Geometry check sheet. Reference: drawing and pictorial views, mm from the part's lowest x, y, z. Give positions to 0.01 mm unless a question says otherwise; leave off trailing zeros. Order: outer loops, then holes, each group sorted by start corner. A loop starts at its lowest first (then second) coordinate and runs counter-clockwise, first axis right, second up. Notation, with made-up numbers: (55, -37.75) - (59, -37.75) arc R19 cw to (59, -9.75) - close; hole circle Ø6 at (48.5, 30). An arc over 180 degrees is marked (long way). Answer as a JSON object with one key per item and string values.
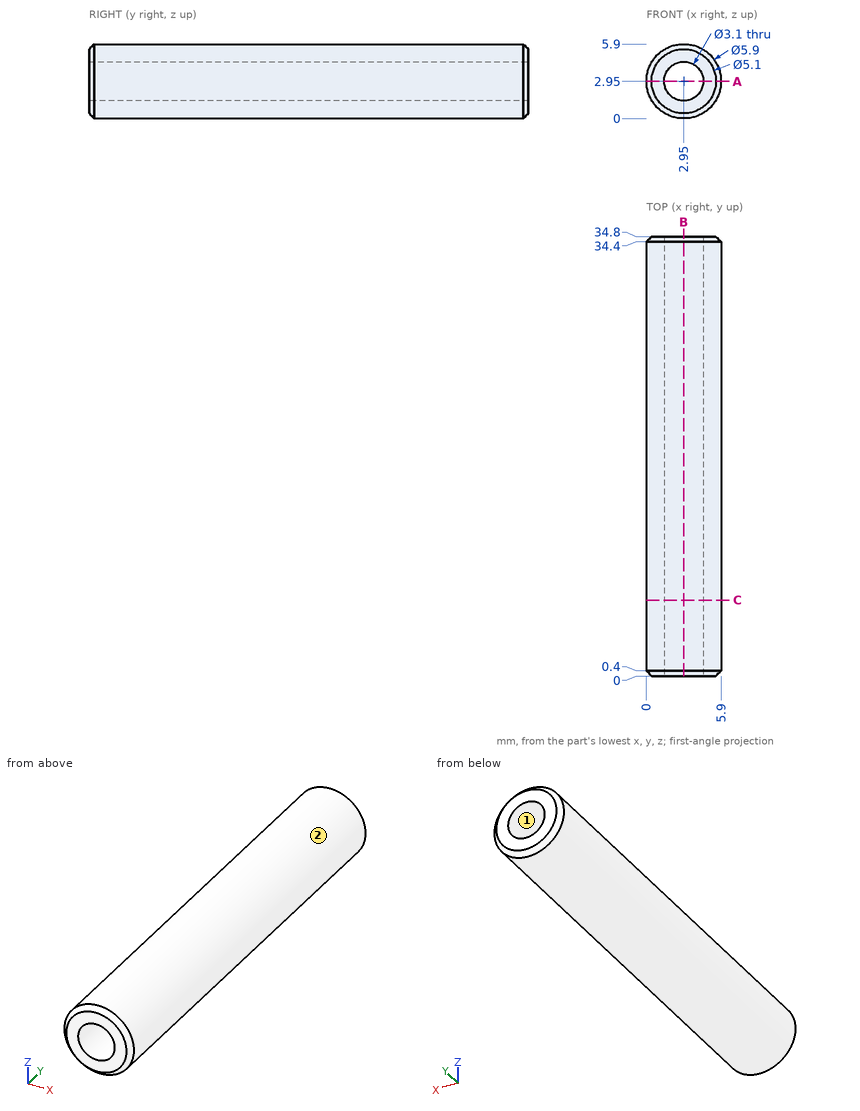
(1) Release check for a two-part mould opening along Z. For the marked faces 1 and 2 record: pulls with the +Z half, pulls with the -Z half, needs draft (parallel to the pull), parting line crosses it, or undercut.
Computed values:
{"face 1": "undercut", "face 2": "parting line crosses it"}
(2) Section check B-B (x = 2.95). Record the cut outline in (y, z), then the cut area to 3 significant figures.
Computed values:
{"outline": "(0, 0.4) - (0.4, 0) - (34.4, 0) - (34.8, 0.4) - (34.8, 1.4) - (0, 1.4) - close; (0, 4.5) - (34.8, 4.5) - (34.8, 5.5) - (34.4, 5.9) - (0.4, 5.9) - (0, 5.5) - close", "area": "97.1 mm²"}
(3) Material ranges on line 1 along X through (y, z) = (10.5, 2.95); line 2 along Z through (x, y) = (3.1, 22); line 3 along Z through (x, y) = (2.1, 18), recorded low to high. Write a range as [from, to].
Computed values:
{"line 1": "x = [0, 1.4], [4.5, 5.9]", "line 2": "z = [0, 1.41], [4.49, 5.9]", "line 3": "z = [0.13, 1.65], [4.25, 5.77]"}
(4) Gauge pin test, flat end, axial feed: pin 1 Ø1 at (x, y) = (4.5, 31) entering from +Z. Record the tip position at first contact, or that the pin passes through.
Computed values:
{"pin 1": "stops at z = 5.71"}
(5) Section check A-A (z = 2.95). Record the cut outline in (x, y).
Computed values:
{"outline": "(0, 0.4) - (0.4, 0) - (1.4, 0) - (1.4, 34.8) - (0.4, 34.8) - (0, 34.4) - close; (4.5, 0) - (5.5, 0) - (5.9, 0.4) - (5.9, 34.4) - (5.5, 34.8) - (4.5, 34.8) - close"}
(6) Section check C-C (y = 6). Record the cut outline in (x, z).
Computed values:
{"outline": "circle Ø5.9 at (2.95, 2.95); hole circle Ø3.1 at (2.95, 2.95)"}
